Autodesk Inventor part; units mm, degrees
ref_plane "YZ Plane" through (0, 0, 0) normal (1, 0, 0) x (0, 1, 0)
ref_plane "XZ Plane" through (0, 0, 0) normal (0, 1, 0) x (-1, 0, 0)
ref_plane "XY Plane" through (0, 0, 0) normal (0, 0, 1) x (1, 0, 0)
sketch "Sketch1" plane through (0, 0, 0) normal (0, 1, 0) x (-1, 0, 0)
  line L0 (0, 108) -> (0, 0)
  line L1 (0, 0) -> (10.412, 0)
  line L2 (10.412, 0) -> (109.1455, 26.4556)
  line L3 (109.1455, 26.4556) -> (109.1455, 81.5444)
  line L4 (109.1455, 81.5444) -> (10.412, 108)
  line L5 (10.412, 108) -> (0, 108)
  line L6 (2.5529, 107) -> (1, 101.2044) construction
  line L7 (1, 101.2044) -> (97.5926, 75.3225) construction
  line L8 (97.5926, 75.3225) -> (99.1455, 81.1181) construction
  line L9 (99.1455, 81.1181) -> (2.5529, 107) construction
  line L10 (1, 6.7956) -> (2.5529, 1) construction
  line L11 (2.5529, 1) -> (99.1455, 26.8819) construction
  line L12 (99.1455, 26.8819) -> (97.5926, 32.6775) construction
  line L13 (97.5926, 32.6775) -> (1, 6.7956) construction
  line L14 (100.1455, 80.5444) -> (106.1455, 80.5444) construction
  line L15 (106.1455, 80.5444) -> (106.1455, 27.4556) construction
  line L16 (106.1455, 27.4556) -> (100.1455, 27.4556) construction
  line L17 (100.1455, 27.4556) -> (100.1455, 80.5444) construction
  line L18 (17.0418, 103.1177) -> (15.4889, 97.3222)
  line L19 (15.4889, 97.3222) -> (23.2163, 95.2516)
  line L20 (23.2163, 95.2516) -> (24.7692, 101.0472)
  line L21 (24.7692, 101.0472) -> (17.0418, 103.1177)
  line L22 (46.9855, 95.0943) -> (45.4326, 89.2988)
  line L23 (45.4326, 89.2988) -> (53.16, 87.2282)
  line L24 (53.16, 87.2282) -> (54.7129, 93.0238)
  line L25 (54.7129, 93.0238) -> (46.9855, 95.0943)
  line L26 (76.9292, 87.0709) -> (75.3763, 81.2754)
  line L27 (75.3763, 81.2754) -> (83.1037, 79.2048)
  line L28 (83.1037, 79.2048) -> (84.6566, 85.0004)
  line L29 (84.6566, 85.0004) -> (76.9292, 87.0709)
  line L30 (15.4889, 10.6778) -> (17.0418, 4.8823)
  line L31 (17.0418, 4.8823) -> (24.7692, 6.9528)
  line L32 (24.7692, 6.9528) -> (23.2163, 12.7484)
  line L33 (23.2163, 12.7484) -> (15.4889, 10.6778)
  line L34 (45.4326, 18.7012) -> (46.9855, 12.9057)
  line L35 (46.9855, 12.9057) -> (54.7129, 14.9762)
  line L36 (54.7129, 14.9762) -> (53.16, 20.7718)
  line L37 (53.16, 20.7718) -> (45.4326, 18.7012)
  line L38 (75.3763, 26.7246) -> (76.9292, 20.9291)
  line L39 (76.9292, 20.9291) -> (84.6566, 22.9996)
  line L40 (84.6566, 22.9996) -> (83.1037, 28.7952)
  line L41 (83.1037, 28.7952) -> (75.3763, 26.7246)
  line L42 (23.9928, 98.1494) -> (46.209, 92.1965) construction
  line L43 (53.9365, 90.126) -> (76.1527, 84.1732) construction
  line L44 (23.9928, 9.8506) -> (46.209, 15.8035) construction
  line L45 (53.9365, 17.874) -> (76.1527, 23.8268) construction
  line L46 (83.8802, 82.1026) -> (98.369, 78.2203) construction
  line L47 (16.2653, 7.7801) -> (1.7765, 3.8978) construction
  line L48 (83.8802, 25.8974) -> (98.369, 29.7797) construction
  line L49 (16.2653, 100.2199) -> (1.7765, 104.1022) construction
  line L50 (100.1455, 72.5444) -> (106.1455, 72.5444)
  line L51 (106.1455, 72.5444) -> (106.1455, 64.5444)
  line L52 (106.1455, 64.5444) -> (100.1455, 64.5444)
  line L53 (100.1455, 64.5444) -> (100.1455, 72.5444)
  line L54 (100.1455, 43.4556) -> (106.1455, 43.4556)
  line L55 (106.1455, 43.4556) -> (106.1455, 35.4556)
  line L56 (106.1455, 35.4556) -> (100.1455, 35.4556)
  line L57 (100.1455, 35.4556) -> (100.1455, 43.4556)
  line L58 (103.1455, 72.5444) -> (103.1455, 80.5444) construction
  line L59 (103.1455, 35.4556) -> (103.1455, 27.4556) construction
  dimension "d0" = 100
  dimension "d1" = 6
  dimension "d3" = 100
  dimension "d4" = 6
  dimension "d7" = 3
  dimension "d8" = 3
  dimension "d9" = 6
  dimension "d10" = 3
  dimension "d11" = 1
  dimension "d12" = 1
  dimension "d13" = 1
  dimension "d14" = 1
  dimension "d15" = 15
  dimension "d16" = 1
  dimension "d17" = 1
  dimension "d18" = 1
  dimension "d19" = 108
  dimension "d20" = 8
  dimension "d21" = 15
  dimension "d22" = 8
extrude "Extrusion1" add sketch "Sketch1" along normal blind 6
sketch "Sketch2" plane through (0, 0, 0) normal (0, -1, 0) x (1, 0, 0)
  line L0 (0, 0) -> (0, 108)
  line L1 (0, 102) -> (4, 102)
  line L2 (6, 100) -> (6, 96)
  line L3 (4, 94) -> (0, 94)
  line L4 (0, 94) -> (0, 102)
  line L5 (0, 58) -> (4, 58)
  line L6 (6, 56) -> (6, 52)
  line L7 (4, 50) -> (0, 50)
  line L8 (0, 50) -> (0, 58)
  line L9 (0, 14) -> (4, 14)
  line L10 (6, 12) -> (6, 8)
  line L11 (4, 6) -> (0, 6)
  line L12 (0, 6) -> (0, 14)
  arc A0 (6, 100) -> (4, 102) centre (4, 100) ccw
  arc A1 (4, 94) -> (6, 96) centre (4, 96) ccw
  arc A2 (6, 56) -> (4, 58) centre (4, 56) ccw
  arc A3 (4, 50) -> (6, 52) centre (4, 52) ccw
  arc A4 (6, 12) -> (4, 14) centre (4, 12) ccw
  arc A5 (4, 6) -> (6, 8) centre (4, 8) ccw
  line L13 (2, 94) -> (2, 58) construction
  line L14 (2, 50) -> (2, 14) construction
  line L15 (0, 108) -> (-10.412, 108)
  point P0 (6, 54)
  point P1 (0, 54)
  dimension "d25" = 2
  dimension "d26" = 6
  dimension "d27" = 8
  dimension "d28" = 8
  dimension "d29" = 8
  dimension "d38" = 6
extrude "Extrusion2" add sketch "Sketch2" against normal blind 6
sketch "Sketch3" plane through (0, 0, 0) normal (0, -1, 0) x (1, 0, 0)
  line L0 (0, 58) -> (0, 94)
  line L1 (0, 108) -> (-10.412, 108)
  line L2 (0, 92) -> (-6, 92)
  line L3 (-6, 92) -> (-6, 76)
  line L4 (-6, 76) -> (0, 76)
  line L5 (0, 76) -> (0, 92)
  dimension "d33" = 16
  dimension "d34" = 6
  dimension "d35" = 16
extrude "Extrusion3" cut sketch "Sketch3" against normal blind 6
sketch "Sketch4" plane through (0, 0, 0) normal (0, -1, 0) x (1, 0, 0)
  line L0 (-10.412, 108) -> (-109.1455, 81.5444)
  line L1 (0, 58) -> (0, 76)
  line L2 (-23.2163, 95.2516) -> (-24.7692, 101.0472)
  line L3 (-56.7165, 71.5226) -> (-56.0695, 69.1077)
  line L4 (-56.0695, 69.1077) -> (-30.9554, 75.837)
  line L5 (-30.9554, 75.837) -> (-31.6024, 78.2519)
  line L6 (-31.6024, 78.2519) -> (-56.7165, 71.5226)
  line L7 (-56.1041, 71.169) -> (-55.7159, 69.7201) construction
  line L8 (-55.7159, 69.7201) -> (-31.5678, 76.1906) construction
  line L9 (-31.5678, 76.1906) -> (-31.956, 77.6395) construction
  line L10 (-31.956, 77.6395) -> (-56.1041, 71.169) construction
  line L11 (-44.1595, 74.8872) -> (-43.5124, 72.4724) construction
  line L12 (-31.2789, 77.0445) -> (-56.393, 70.3152) construction
  point P0 (-44.0301, 74.4042)
  point P1 (-31.7619, 76.915)
  dimension "d39" = 26
  dimension "d41" = 2.5
  dimension "d43" = 1.5
  dimension "d44" = 25
  dimension "d45" = 31.956
  dimension "d48" = 23.75
extrude "Extrusion4" cut sketch "Sketch4" against normal through all
chamfer "Chamfer1" distance 2 angle 45 2 edges at (-109.1455, 3, 81.5444) (-109.1455, 3, 26.4556)
sketch "Sketch5" plane through (0, 0, 0) normal (0, -1, 0) x (1, 0, 0)
  line L0 (-83.1037, 79.2048) -> (-84.6566, 85.0004)
  circle A0 centre (-88.9513, 80.7438) radius 2.25
  line L1 (-88.9513, 80.7438) -> (-83.8802, 82.1026) construction
  line L2 (-106.1455, 64.5444) -> (-100.1455, 43.4556) construction
  line L3 (-106.1455, 43.4556) -> (-100.1455, 64.5444) construction
  line L4 (-75.3763, 26.7246) -> (-54.7129, 14.9762) construction
  line L5 (-53.16, 20.7718) -> (-76.9292, 20.9291) construction
  line L6 (-45.4326, 18.7012) -> (-24.7692, 6.9528) construction
  line L7 (-46.9855, 12.9057) -> (-23.2163, 12.7484) construction
  circle A1 centre (-103.1455, 54) radius 2.25
  circle A2 centre (-65.0446, 20.8504) radius 2.25
  circle A3 centre (-35.1009, 12.827) radius 2.25
  dimension "d52" = 5.25
  dimension "d53" = 4.5
extrude "Extrusion5" cut sketch "Sketch5" against normal through all
sketch "Sketch6" plane through (0, 0, 0) normal (0, -1, 0) x (1, 0, 0)
  line L0 (0, 14) -> (0, 50)
  line L1 (4, 58) -> (0, 58)
  line L2 (0, 58) -> (0, 76)
  line L3 (0, 68.25) -> (0, 63.75)
  line L4 (-16.3, 63.75) -> (-16.3, 68.25)
  line L5 (-12.3, 70.75) -> (-5, 70.75)
  line L6 (-5, 61.25) -> (-12.3, 61.25)
  line L7 (-16.3, 68.25) -> (-12.3, 68.25)
  line L8 (-5, 68.25) -> (0, 68.25)
  line L9 (0, 63.75) -> (-5, 63.75)
  line L10 (-12.3, 63.75) -> (-16.3, 63.75)
  line L11 (-12.3, 61.25) -> (-12.3, 63.75)
  line L12 (-12.3, 68.25) -> (-12.3, 70.75)
  line L13 (-5, 70.75) -> (-5, 68.25)
  line L14 (-5, 63.75) -> (-5, 61.25)
  line L15 (0, 34.25) -> (0, 29.75)
  line L16 (-16.3, 29.75) -> (-16.3, 34.25)
  line L17 (-12.3, 36.75) -> (-5, 36.75)
  line L18 (-5, 27.25) -> (-12.3, 27.25)
  line L19 (-16.3, 34.25) -> (-12.3, 34.25)
  line L20 (-5, 34.25) -> (0, 34.25)
  line L21 (0, 29.75) -> (-5, 29.75)
  line L22 (-12.3, 29.75) -> (-16.3, 29.75)
  line L23 (-12.3, 27.25) -> (-12.3, 29.75)
  line L24 (-12.3, 34.25) -> (-12.3, 36.75)
  line L25 (-5, 36.75) -> (-5, 34.25)
  line L26 (-5, 29.75) -> (-5, 27.25)
  point P0 (0, 32)
  point P1 (-16.3, 66)
  dimension "d56" = 4.5
  dimension "d57" = 2.5
  dimension "d58" = 2.5
  dimension "d59" = 4
  dimension "d60" = 5
  dimension "d61" = 7.3
  dimension "d62" = 4.5
  dimension "d63" = 2.5
  dimension "d64" = 2.5
  dimension "d65" = 4
  dimension "d66" = 5
  dimension "d67" = 7.3
  dimension "d68" = 8
extrude "Extrusion6" cut sketch "Sketch6" against normal through all
equation "\"d3\" = d0"
equation "\"d4\" = d1"
equation "\"d8\" = d7"
equation "\"d9\" = d1"
equation "\"d10\" = d7"
equation "\"d12\" = d11"
equation "\"d28\" = d27"
equation "\"d29\" = d28"
equation "\"d58\" = d57"
equation "\"d64\" = d63"
properties part number "front_panel_2004_brace"
Geometry: final body of the model. Coordinates: model frame, mm. A direction names the side the tool comes from. Give positions to 0.01 mm unless a question says otherwise; leave off trailing zeros. Order: outer loops, then holes, each group sorted by start corner. A loop starts at its lowest first (then second) coordinate and runs counter-clockwise, first axis right, second up. Notation, with made-up numbers: (39, 51) -> (79, 51) arc R15 ccw to (79, 60) -> close; hole circle Ø8 at (-38, 79). An arc over 180 degrees is marked (long way). Write each question's results on one line, items separated by ' | '. Start each with the question number.
1) Draft query along Z for faces 1 (the flat face through (-109.146, 3, 54)), 2 (the flat face through (2, 3, 6)), 3 (the flat face through (0, 3, 22)). Return one class per face: pulls with the +Z half, pulls with the -Z half, needs draft (parallel to the pull), parting line crosses it, or undercut.
2) Set-up query: faces 4 (the flat face through (-9, 3, 27.25)), 5 (the flat face through (2, 3, 102)), 6 (the flat face through (-51, 6, 55)), 7 (the flat face through (-14, 3, 34.25)). Return all of +Z, -Z, +X, -X, +Y, -Y with unobstructed straight access to the full face (end or side cutting, diameter ignored); none if empty.
3) First-contact query: pin 1 (2 mm diameter, centred on x = -16.5, y = 1.5, fed in from +Z); pin 2 (3 mm diameter, centred on y = 2, z = 1.5, fed in from +X); pin 3 (2 mm diameter, centred on x = 2.5, y = 3, fed in from -Z). Flat tips, straight axial feed; report the tip coordinate or a pass-through.
4) Line query: line 1 (Z direction, x = -1, y = 3.2); line 2 (Z direction, x = -8.5, y = 3.45); line 3 (X direction, y = 2.5, z = 67.5). Output: solid intervals per line, ascending. Write a range as from..to.
5) Section A-A (z = 41). Return loops of the section in (x, y), then the cut area to 3 significant figures.
6) Section C-C (x = -98). Return loops of the section in (y, z), then the cut area to 3 significant figures.
7) Section B-B (x = -41.5). Return loops of the section in (y, z), then the cut area to 3 significant figures.
8) Section D-D (y = 1.35). Count the separate pieces of the cut face and the enclosed holes in it, then the cut area to 3 significant figures.
Calculated:
1) face 1: needs draft | face 2: pulls with the -Z half | face 3: undercut
2) face 4: +Y, -Y | face 5: +Z, +X, +Y, -Y | face 6: +Z, -Z, +X, -X, +Y | face 7: +X, +Y, -Y
3) pin 1: z = 106.64 | pin 2: x = 0 | pin 3: z = 6
4) line 1: 0..29.75, 34.25..63.75, 68.25..76, 92..108 | line 2: 0..27.25, 36.75..61.25, 70.75..108 | line 3: -109.15..-106.15, -100.15..-16.3
5) outline: (-109.15, 0) -> (-106.15, 0) -> (-106.15, 6) -> (-109.15, 6) -> close; (-100.15, 0) -> (0, 0) -> (0, 6) -> (-100.15, 6) -> close | area: 619 mm2
6) outline: (0, 23.47) -> (6, 23.47) -> (6, 84.53) -> (0, 84.53) -> close | area: 366 mm2
7) outline: (0, 8.33) -> (6, 8.33) -> (6, 73.01) -> (0, 73.01) -> close; (0, 75.6) -> (6, 75.6) -> (6, 99.67) -> (0, 99.67) -> close | area: 533 mm2
8) separate pieces: 1 | enclosed holes: 13 | area: 8,480 mm2
